Build history of the part. All positions in model axes, mm. Give positions to 0.01 mm unless a question says otherwise; leave off trailing zeros. Order: outer loops, then holes, each group sorted by start corner. A loop starts at its lowest first (then second) coordinate and runs counter-clockwise, first axis right, second up. Notation, with made-up numbers: (35.5, 75) - (73.5, 75) arc R19 cw to (73.5, 94) - close; hole circle Ø1 at (-37.5, 64.25). An arc over 180 degrees is marked (long way). Use a Markdown table: item, result. Add a question column.
(1) Slice it at B-B (y = -1.5). Write the cut outline in (x, z).
(2) Slice it at C-C (z = -63). Write the cut outline in (x, y), then the cut area to 3 significant figures.
(3) Slice it at A-A (x = -67.5). Write the cut outline in (y, z).
(4) Wall check: line 1 (Z direction, x = 114.5, y = -2.5); line 2 (Z direction, x = 32, y = -1.5); line 3 (Y direction, x = -8, z = -71.5). Give the ranges that are in metal, low to high.
from build123d import *

# Parameters (mm, degrees)
F0_W     = 300
F0_H     = 100
F1_DEPTH = 9
F3_DEPTH = 300.001


with BuildPart() as f1:
    # F0 (on Front) → F1 (new body, symmetric)
    with BuildSketch(Plane.XZ):
        with Locations((-3.72486, -105.77762)):
            Rectangle(F0_W, F0_H)
    extrude(amount=F1_DEPTH, both=True)

    # F2 (on face) → F3 (cut, through all)
    with BuildSketch(Plane.YZ.offset(146.27514)):
        Polygon((-9, -55.77762), (-9, -75.77762), (2.547005, -55.77762), align=None)
    extrude(amount=-F3_DEPTH, mode=Mode.SUBTRACT)


solid = f1.part
Solution:
| question | item | result |
|---|---|---|
| 1 | outline | (-153.72, -155.78) - (146.28, -155.78) - (146.28, -62.79) - (-153.72, -62.79) - close |
| 2 | outline | (-153.72, -1.62) - (146.28, -1.62) - (146.28, 9) - (-153.72, 9) - close |
| 2 | area | 3,190 mm2 |
| 3 | outline | (-9, -155.78) - (9, -155.78) - (9, -55.78) - (2.55, -55.78) - (-9, -75.78) - close |
| 4 | line 1 | -155.78 to -64.52 |
| 4 | line 2 | -155.78 to -62.79 |
| 4 | line 3 | -6.53 to 9 |
